Here's how the part is built. I have some questions about the finished solid (model axes, mm). Face numbers are marked on the shaded views. A direction names the side the tool comes from. Coordinates: 2 decimals unless noted, no trailing zeros. Write each loop counter-clockwise with the first axis right and the second up, starting at its lowest first coordinate (ties: lowest second). Pieces come first, ordered by that corner, then holes.
(1) Imagine slicing it at C-C, the plane y = 18. List the corners of the cut face in (x, z) for me.
(2) Please list where these lines run through material, in increasing order: probe 1 along Y at (x, z) = (22.5, 7.25); probe 2 along X at (y, z) = (37.5, 3.25); probe 3 along Z at (x, y) = (-19, 40).
(3) Which directions (+Z, -Z, +X, -X, +Y, -Y) give clear straight access to the entire face, cutting with the end or side of a thin tool? Please do the marked faces 1, 2 and 3.
(4) Imagine slicing it at B-B, the plane z = 5.75. List the corners of the cut face in (x, y) for me.
(5) Imagine slicing it at A-A, the plane x = -17.5. List the corners of the cut face in (y, z) for me, plus the area to 3 significant figures.
(6) For pin 1 Ø3.5 at (x, z) = (-21, 5) entering from +Y; pin 2 Ø6 at (x, y) = (-14.5, 43) entering from +Z; pin 3 Ø2.5 at (y, z) = (38.5, 3.5) entering from -X, each with a flat end and sliding along its axis, tell me the tip position at first contact or that it passes through.
(7) Imagine slicing it at D-D, the plane x = -2. List the corners of the cut face in (y, z) for me.
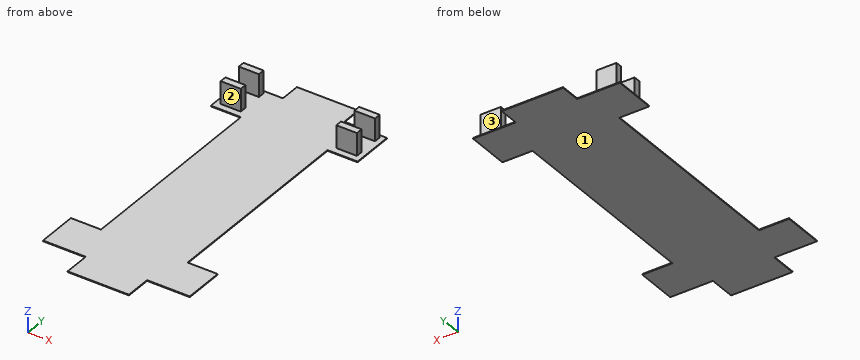
```python
from build123d import *

# Parameters (mm, degrees)
F1_DEPTH = 0.254
F2_W     = 6.786758
F2_H     = 2.286
F2_W_2   = 6.9342
F3_DEPTH = 7.62


with BuildPart() as f1:
    # F0 (on Top) → F1 (new body)
    with BuildSketch(Plane.XY):
        Polygon((-10.351698, -56.194937), (10.351697, -56.194937), (10.351697, -47.322049), (24.770136, -47.322049), (24.770136, -33.643018), (14.610136, -33.643018), (14.610136, 34.936982), (24.770136, 34.936982), (24.770136, 49.355418), (10.351697, 49.355418), (10.351697, 56.194937), (-10.351698, 56.194937), (-10.351698, 49.355418), (-24.770136, 49.355418), (-24.770136, 34.936982), (-14.610136, 34.936982), (-14.610136, -33.643018), (-24.770136, -33.643018), (-24.770136, -47.322049), (-10.351698, -47.322049), align=None)
    extrude(amount=-F1_DEPTH)

    # F2 (on face) → F3 (join)
    with BuildSketch(Plane.XY):
        with Locations((-19.598757, 47.214477)):
            Rectangle(F2_W, F2_H)
        with Locations((-19.598757, 38.324477)):
            Rectangle(F2_W, F2_H)
        with Locations((19.525036, 38.324478)):
            Rectangle(F2_W_2, F2_H)
        with Locations((19.525036, 47.214478)):
            Rectangle(F2_W_2, F2_H)
    extrude(amount=F3_DEPTH)


solid = f1.part
```
Recorded:
1. outline: (-14.61, -0.25) - (14.61, -0.25) - (14.61, 0) - (-14.61, 0) - close
2. probe 1: y = 37.18 to 39.47, 46.07 to 48.36
2. probe 2: x = -22.99 to -16.21, 16.06 to 22.99
2. probe 3: z = -0.25 to 0
3. face 1: -Z, +X, -X, +Y, -Y
3. face 2: +Z, +X, -X, -Y
3. face 3: +Z, +X, -X, +Y
4. outline: (-22.99, 37.18) - (-16.21, 37.18) - (-16.21, 39.47) - (-22.99, 39.47) - close; (-22.99, 46.07) - (-16.21, 46.07) - (-16.21, 48.36) - (-22.99, 48.36) - close; (16.06, 37.18) - (22.99, 37.18) - (22.99, 39.47) - (16.06, 39.47) - close; (16.06, 46.07) - (22.99, 46.07) - (22.99, 48.36) - (16.06, 48.36) - close
5. outline: (-47.32, -0.25) - (-33.64, -0.25) - (-33.64, 0) - (-47.32, 0) - close; (34.94, -0.25) - (49.36, -0.25) - (49.36, 0) - (48.36, 0) - (48.36, 7.62) - (46.07, 7.62) - (46.07, 0) - (39.47, 0) - (39.47, 7.62) - (37.18, 7.62) - (37.18, 0) - (34.94, 0) - close
5. area: 42.0 mm2
6. pin 1: stops at y = 48.36
6. pin 2: stops at z = 0
6. pin 3: stops at x = -22.99
7. outline: (-56.19, -0.25) - (56.19, -0.25) - (56.19, 0) - (-56.19, 0) - close
